For this review, take the finished solid that the model builds, in its own axes (mm). Face numbers are marked on the shaded views. Coordinates: 2 decimals unless noted, no trailing zeros. Order: outer loops, then holes, each group sorted by start corner. A loop starts at its lowest first (then second) coordinate and runs counter-clockwise, first axis right, second up.
from build123d import *

# Parameters (mm, degrees)
F1_DEPTH = 500
F3_DEPTH = 80
F5_DEPTH = 80.001


# Not quite as in the source:
# - a pattern or mirror of a feature is missing from the dataset's text; its kind, count and spacing are read off the source's solid


with BuildPart() as f1:
    # F0 (on Right) → F1 (new body, symmetric)
    with BuildSketch(Plane.YZ):
        with BuildLine():
            Line((35, 40), (-35, 40))
            ThreePointArc((-35, 40), (-38.5355339059, 38.5355339059), (-40, 35))
            Line((-40, 35), (-40, -35))
            ThreePointArc((-40, -35), (-38.5355339059, -38.5355339059), (-35, -40))
            Line((-35, -40), (35, -40))
            ThreePointArc((35, -40), (38.5355339059, -38.5355339059), (40, -35))
            Line((40, -35), (40, 35))
            ThreePointArc((40, 35), (38.5355339059, 38.5355339059), (35, 40))
        make_face()
        with BuildLine():
            ThreePointArc((-36, 32), (-34.8284271247, 34.8284271247), (-32, 36))
            Line((-32, 36), (32, 36))
            ThreePointArc((32, 36), (34.8284271247, 34.8284271247), (36, 32))
            Line((36, 32), (36, -32))
            ThreePointArc((36, -32), (34.8284271247, -34.8284271247), (32, -36))
            Line((32, -36), (-32, -36))
            ThreePointArc((-32, -36), (-34.8284271247, -34.8284271247), (-36, -32))
            Line((-36, -32), (-36, 32))
        make_face(mode=Mode.SUBTRACT)
    extrude(amount=F1_DEPTH, both=True)

    # F2 (on face) → F3 (cut, through all)
    with BuildSketch(Plane.XY.offset(40)):
        Polygon((-500, 30.4411906294), (-540, 45), (-540, -54.9271104923), (-265.4525203311, -54.9271104923), (-320.2018064436, -35), (-500, -35), align=None)
        Polygon((-320.2018064436, -35), (-500, 30.4411906294), (-500, -35), align=None)
    f3 = extrude(amount=-F3_DEPTH, mode=Mode.SUBTRACT)

    # F3_copies: F3 across plane
    add(f3.mirror(Plane(origin=(0, 0, 0), x_dir=(0, 0, 1), z_dir=(1, 0, 0))), mode=Mode.SUBTRACT)

    # F4 (on face) → F5 (cut, through all)
    with BuildSketch(Plane.XY.offset(40)):
        with BuildLine():
            Line((100, 0), (200, 0))
            ThreePointArc((200, 0), (210, 10), (200, 20))
            Line((200, 20), (100, 20))
            ThreePointArc((100, 20), (90, 10), (100, 0))
        make_face()
    extrude(amount=-F5_DEPTH, mode=Mode.SUBTRACT)


solid = f1.part
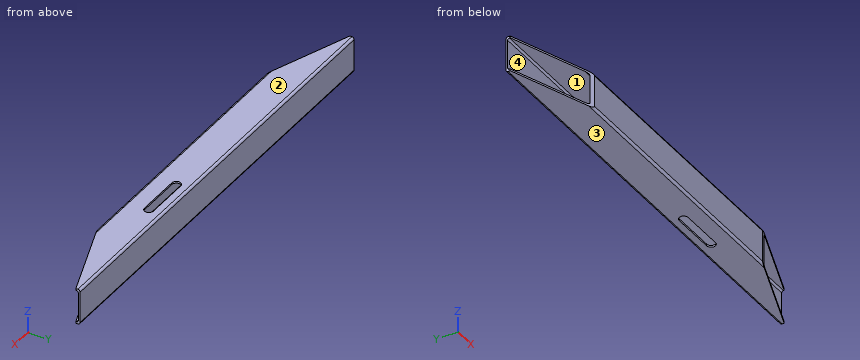
1. Clearance check with flat-ended pins moving along their axes: pin 1 Ø2 at (x, z) = (148, -39) entering from -Y; pin 2 Ø1.2 at (x, z) = (157, 37.5) entering from -Y; pin 3 Ø3 at (x, z) = (140, 39) entering from +Y. State where each tip first meets the part, or that it passes through.
Answer below:
pin 1: stops at y = -39
pin 2: stops at y = -39.62
pin 3: stops at y = 39.33
2. Take a section at B-B, the plane x = 282. Give the boundary of the cut face in (y, z).
Answer below:
outline: (-40, -35) arc R5 ccw to (-35, -40) - (35, -40) arc R5 ccw to (40, -35) - (40, 35) arc R5 ccw to (35, 40) - (-35, 40) arc R5 ccw to (-40, 35) - close; hole (-36, -32) arc R4 ccw to (-32, -36) - (32, -36) arc R4 ccw to (36, -32) - (36, 32) arc R4 ccw to (32, 36) - (-32, 36) arc R4 ccw to (-36, 32) - close
3. Take a section at D-D, the plane x = -420. Give the boundary of the cut face in (y, z), plus the area to 3 significant figures.
Answer below:
outline: (1.32, -40) - (35, -40) arc R5 ccw to (40, -35) - (40, 35) arc R5 ccw to (35, 40) - (1.32, 40) - (1.32, 36) - (32, 36) arc R4 cw to (36, 32) - (36, -32) arc R4 cw to (32, -36) - (1.32, -36) - close
area: 594 mm2
4. To check wall thickness, follow L1, parallel to Y at x = -158, z = -10.5; L2, parallel to Z at x = -106, y = 34.5. State the ranges of each line that lie inside material, in increasing order.
Answer below:
L1: y = -40 to -36, 36 to 40
L2: z = -40 to -35.12, 35.12 to 40
5. The part is to be moulded in two halves that separate along Z. For the marked faces 1, 2, 3 and 4, say which applies: +Z half, -Z half, draft (parallel to the pull), parting line (faces both ways), or undercut.
Answer below:
face 1: undercut
face 2: +Z half
face 3: -Z half
face 4: undercut
6. Take a section at A-A, the plane z = 16. Give the boundary of the cut face in (x, y), plus the area to 3 significant figures.
Answer below:
outline: (-500, 36) - (500, 36) - (500, 40) - (-500, 40) - close; (-317.45, -36) - (-306.46, -40) - (306.46, -40) - (317.45, -36) - close
area: 6,500 mm2
7. Take a section at C-C, the plane y = 10. Give the boundary of the cut face in (x, z).
Answer below:
outline: (-443.84, -40) - (90, -40) - (90, -36) - (-443.84, -36) - close; (-443.84, 36) - (90, 36) - (90, 40) - (-443.84, 40) - close; (210, -40) - (443.84, -40) - (443.84, -36) - (210, -36) - close; (210, 36) - (443.84, 36) - (443.84, 40) - (210, 40) - close
